```python
from build123d import *

# Parameters (mm, degrees)
SKETCH_1_W               = 60
SKETCH_1_H               = 100
SKETCH_1_R               = 4
SKETCH_1_R_2             = 2
EXTRUDE_1_DEPTH          = 19
SKETCH_3_W               = 20
SKETCH_3_H               = 50
SKETCH_3_H_2             = 10
SKETCH_3_W_2             = 10
SKETCH_3_H_3             = 20
CUT_EXTRUDE_1_DEPTH      = 62.326992426
CHAMFER_1_SIZE           = 3
CUT_EXTRUDE_2_DEPTH      = 62.326992426
CUT_EXTRUDE_2_DEPTH_BACK = 62.326992426


with BuildPart() as part:
    # 草图1 → 凸台-拉伸1 (new body)
    with BuildSketch(Plane(origin=(0, 0, 0), x_dir=(1, 0, 0), z_dir=(0, 1, 0))):
        Rectangle(SKETCH_1_W, SKETCH_1_H)
        with Locations(Location((-20, 0, 0), (0, 0, 270))):
            Circle(SKETCH_1_R, mode=Mode.SUBTRACT)
        with Locations(Location((20, 0, 0), (0, 0, 270))):
            Circle(SKETCH_1_R, mode=Mode.SUBTRACT)
        with Locations(Location((-20, -40, 0), (0, 0, 270))):
            Circle(SKETCH_1_R, mode=Mode.SUBTRACT)
        with Locations(Location((20, -40, 0), (0, 0, 270))):
            Circle(SKETCH_1_R, mode=Mode.SUBTRACT)
        with Locations(Location((-20, 40, 0), (0, 0, 270))):
            Circle(SKETCH_1_R, mode=Mode.SUBTRACT)
        with Locations(Location((20, 40, 0), (0, 0, 270))):
            Circle(SKETCH_1_R, mode=Mode.SUBTRACT)
        with Locations(Location((-9, -30, 0), (0, 0, 270))):
            Circle(SKETCH_1_R_2, mode=Mode.SUBTRACT)
        with Locations(Location((9, -30, 0), (0, 0, 270))):
            Circle(SKETCH_1_R_2, mode=Mode.SUBTRACT)
        with Locations(Location((-9, -10, 0), (0, 0, 270))):
            Circle(SKETCH_1_R_2, mode=Mode.SUBTRACT)
        with Locations(Location((9, -10, 0), (0, 0, 270))):
            Circle(SKETCH_1_R_2, mode=Mode.SUBTRACT)
    extrude(amount=EXTRUDE_1_DEPTH)

    # 草图3 → 切除-拉伸1 (cut, through all)
    with BuildSketch(Plane(origin=(0, 0, 0), x_dir=(1, 0, 0), z_dir=(0, 1, 0))):
        with Locations((0, 25)):
            Rectangle(SKETCH_3_W, SKETCH_3_H)
        with Locations((0, -45)):
            Rectangle(SKETCH_3_W, SKETCH_3_H_2)
        with Locations((-25, -20)):
            Rectangle(SKETCH_3_W_2, SKETCH_3_H_3)
        with Locations((25, -20)):
            Rectangle(SKETCH_3_W_2, SKETCH_3_H_3)
    extrude(amount=CUT_EXTRUDE_1_DEPTH, mode=Mode.SUBTRACT)

    # 倒角1
    chamfer_1_edges = [part.edges().sort_by_distance(p)[0] for p in [
        (-10, 9.5, -50),
        (-10, 9.5, 0),
        (10, 9.5, 0),
        (10, 9.5, -50),
        (-30, 9.5, -50),
        (30, 9.5, -50),
        (-10, 9.5, 40),
        (-10, 9.5, 50),
        (30, 9.5, 50),
        (10, 9.5, 50),
        (10, 9.5, 40),
        (-30, 9.5, 50),
        (-30, 9.5, 10),
        (-30, 9.5, 30),
        (-20, 9.5, 30),
        (-20, 9.5, 10),
        (30, 9.5, 30),
        (30, 9.5, 10),
        (20, 9.5, 10),
        (20, 9.5, 30),
    ]]
    chamfer(chamfer_1_edges, length=CHAMFER_1_SIZE)

    # 草图4 → 切除-拉伸2 (cut, two sides: drawn at the far end of the back side and taken through both)
    with BuildSketch(Plane(origin=(0, 0, 0), x_dir=(0, 0, -1), z_dir=(1, 0, 0)).offset(-CUT_EXTRUDE_2_DEPTH_BACK)):
        Polygon((15, 19), (32, 9), (50, 9), (50, 19), align=None)
    extrude(amount=CUT_EXTRUDE_2_DEPTH + CUT_EXTRUDE_2_DEPTH_BACK, mode=Mode.SUBTRACT)


solid = part.part
```
Part model, mm, in its own coordinate system. A direction names the side the tool comes from. Round coordinates to 2 decimals unless told otherwise and drop trailing zeros. Loops run counter-clockwise (first coordinate to the right, second up) from the corner with the lowest first, then second, coordinate; pieces in that order, holes last.
Item 1: Drop flat-ended pins along their axis: P1, Ø4, axis at x = 2.5, y = 11, coming from the +Z side; P2, Ø2, axis at x = -24.5, y = 12, coming from the -Z side; P3, Ø1, axis at y = 13, z = 16.5, coming from the -X side; P4, Ø2, axis at x = -3.5, z = -2.5, coming from the -Y side. Give the stop position or say it passes through.
Item 2: Drill centre lines: line 1 (X direction, y = 2.5, z = -40); line 2 (Z direction, x = 22.5, y = 14.5); line 3 (Z direction, x = 16.5, y = 4.75). Where is each one in solid material? Low to high.
Item 3: Cut at C-C, the plane x = -17. Give the cut face in (y, z), then the cut area to 3 significant figures.
Item 4: Cut at A-A, the plane x = -9. Give the cut face in (y, z), then the cut area to 3 significant figures.
Item 5: Mould opens along X. For faces 6 (the face through (-30, 9, 40)), 7 (the face through (-11, 9, 48)), 8 (the face through (-20, 9, 50)), 9 (the face through (28, 9, 9)) say: +X half, -X half, draft (parallel to the pull), parting line (faces both ways), or undercut.
Item 6: 3-axis set-ups, long thin cutter, end or side, ignore diameter. For faces 1 (the face through (-20, 9, -45)), 2 (the face through (0, 9, 40)), 3 (the face through (22.7, 4.44, -42.95)), 4 (the face through (20, 9, 50)), 5 (the face through (25, 9, 10)): which of +Z, -Z, +X, -X, +Y, -Y reach the whole face in a straight line?
Item 7: Cut at D-D, the plane y = 14.5. State how many separate pieces and enclosed holes the cut face has, then the cut area to 3 significant figures.
Item 8: Cut at B-B, the plane z = -40. Give the cut face in (x, y), then the cut area to 3 significant figures.
A:
1. P1: stops at z = 40
1. P2: stops at z = -28.6
1. P3: stops at x = -20
1. P4: passes through
2. line 1: x = -30 to -24, -16 to -10, 10 to 16, 24 to 30
2. line 2: z = -22.65 to -3.12, 3.12 to 10.5, 29.5 to 36.88, 43.12 to 50
2. line 3: z = -50 to -41.94, -38.06 to -1.94, 1.94 to 38.06, 41.94 to 50
3. outline: (0, -50) - (9, -50) - (9, -42.65) - (0, -42.65) - close; (0, -37.35) - (9, -37.35) - (9, -32) - (19, -15) - (19, -2.65) - (0, -2.65) - close; (0, 2.65) - (19, 2.65) - (19, 37.35) - (0, 37.35) - close; (0, 42.65) - (19, 42.65) - (19, 50) - (0, 50) - close
3. area: 1,390 mm2
4. outline: (0, -2) - (19, -2) - (19, 8) - (0, 8) - close; (0, 12) - (19, 12) - (19, 28) - (0, 28) - close; (0, 32) - (19, 32) - (19, 42) - (0, 42) - close
4. area: 684 mm2
5. face 6: -X half
5. face 7: undercut
5. face 8: draft
5. face 9: +X half
6. face 1: -Z, +X, -X, +Y
6. face 2: +Z, +Y, -Y
6. face 3: +Y, -Y
6. face 4: +Z, +X, -X, +Y, -Y
6. face 5: +X, +Y, -Y
7. separate pieces: 1
7. enclosed holes: 8
7. area: 3,050 mm2
8. outline: (-30, 0) - (-24, 0) - (-24, 9) - (-30, 9) - close; (-16, 0) - (-10, 0) - (-10, 9) - (-16, 9) - close; (10, 0) - (16, 0) - (16, 9) - (10, 9) - close; (24, 0) - (30, 0) - (30, 9) - (24, 9) - close
8. area: 216 mm2
